Geometry: final body of the model. Coordinates: model frame, mm. A direction names the side the tool comes from. Coordinates: 2 decimals unless noted, no trailing zeros. Write each loop counter-clockwise with the first axis right and the second up, starting at its lowest first coordinate (ties: lowest second). Pieces come first, ordered by that corner, then holes.
from build123d import *

# Parameters (mm, degrees)
F0_W        = 2.5
F0_H        = 3.1
F0_W_2      = 3.1
F0_H_2      = 2.5
F1_DEPTH    = 15
F2_DEPTH    = 0.6
F3_T1_DEPTH = 15


# Not quite as in the source:
# - a fillet or chamfer that OpenCascade refuses, or shapes differently, is made with other operations: its cross-section is extruded or revolved along the edge and cut away or added


with BuildPart() as f1:
    # F0 (on Top) → F1 (new body)
    with BuildSketch(Plane.XY):
        with BuildLine():
            Line((39.1167589883, 43.6909709372), (38.9183741482, 43.5764333963))
            ThreePointArc((38.9183741482, 43.5764333963), (39.563732113, 42.8018800146), (40.1167589265, 41.9589202367))
            Line((40.1167589265, 41.9589202367), (39.1167589883, 43.6909709372))
        make_face()
        with BuildLine():
            ThreePointArc((40.1167589265, -41.8145826694), (39.563732113, -42.6575424473), (38.9183741482, -43.432095829))
            Line((38.9183741482, -43.432095829), (39.1167589883, -43.5466333699))
            Line((39.1167589883, -43.5466333699), (40.1167589265, -41.8145826694))
        make_face()
        with BuildLine():
            Line((41.1167589883, 40.226869322), (40.1167589265, 41.9589202367))
            ThreePointArc((40.1167589265, 41.9589202367), (40.5702701762, 41.0585049774), (40.9183741482, 40.1123317812))
            Line((40.9183741482, 40.1123317812), (41.1167589883, 40.226869322))
        make_face()
        with BuildLine():
            Line((41.1167589883, -40.0825317547), (40.9183741482, -39.9679942139))
            ThreePointArc((40.9183741482, -39.9679942139), (40.5702701762, -40.9141674102), (40.1167589265, -41.8145826694))
            Line((40.1167589265, -41.8145826694), (41.1167589883, -40.0825317547))
        make_face()
        with BuildLine():
            Line((38.9183741482, 43.5764333963), (23.9946357527, 34.9602090164))
            ThreePointArc((23.9946357527, 34.9602090164), (24.7962509126, 33.113620668), (25.9946357527, 31.4961074012))
            Line((25.9946357527, 31.4961074012), (40.9183741482, 40.1123317812))
            ThreePointArc((40.9183741482, 40.1123317812), (40.5702701762, 41.0585049774), (40.1167589265, 41.9589202367))
            ThreePointArc((40.1167589265, 41.9589202367), (39.563732113, 42.8018800146), (38.9183741482, 43.5764333963))
        make_face()
        with BuildLine():
            ThreePointArc((25.9946357527, -31.3517698339), (24.7962509126, -32.9692831007), (23.9946357527, -34.8158714491))
            Line((23.9946357527, -34.8158714491), (38.9183741482, -43.432095829))
            ThreePointArc((38.9183741482, -43.432095829), (39.563732113, -42.6575424473), (40.1167589265, -41.8145826694))
            ThreePointArc((40.1167589265, -41.8145826694), (40.5702701762, -40.9141674102), (40.9183741482, -39.9679942139))
            Line((40.9183741482, -39.9679942139), (25.9946357527, -31.3517698339))
        make_face()
        with BuildLine():
            Line((23.9946357527, 34.9602090164), (-12.8447652387, 13.6909709372))
            Line((-12.8447652387, 13.6909709372), (-20.6597652387, 27.2269479983))
            ThreePointArc((-20.6597652387, 27.2269479983), (-36.3375843281, 0.0721687836), (-20.6597652387, -27.082610431))
            Line((-20.6597652387, -27.082610431), (-12.8447652387, -13.5466333699))
            Line((-12.8447652387, -13.5466333699), (23.9946357527, -34.8158714491))
            ThreePointArc((23.9946357527, -34.8158714491), (24.7962509126, -32.9692831007), (25.9946357527, -31.3517698339))
            Line((25.9946357527, -31.3517698339), (25.7962509126, -31.2372322931))
            Line((25.7962509126, -31.2372322931), (25.7962509126, 31.3815698604))
            Line((25.7962509126, 31.3815698604), (25.9946357527, 31.4961074012))
            ThreePointArc((25.9946357527, 31.4961074012), (24.7962509126, 33.113620668), (23.9946357527, 34.9602090164))
        make_face()
        Polygon((-7.648612816, -11.9278312164), (-7.648612816, 12.0721687836), (21.7962509126, 29.0721687836), (21.7962509126, -28.9278312164), align=None, mode=Mode.SUBTRACT)
        Polygon((-17.998612816, 7.6721687836), (-11.648612816, 7.6721687836), (-11.648612816, 1.3221687836), (-11.648612816, -1.1778312164), (-11.648612816, -7.5278312164), (-17.998612816, -7.5278312164), (-20.498612816, -7.5278312164), (-26.848612816, -7.5278312164), (-26.848612816, -1.1778312164), (-26.848612816, 1.3221687836), (-26.848612816, 7.6721687836), (-20.498612816, 7.6721687836), align=None, mode=Mode.SUBTRACT)
        with Locations((-19.248612816, -5.9778312164)):
            Rectangle(F0_W, F0_H)
        with Locations((-13.198612816, 0.0721687836)):
            Rectangle(F0_W_2, F0_H_2)
        with Locations((-19.248612816, 6.1221687836)):
            Rectangle(F0_W, F0_H)
        with Locations((-25.298612816, 0.0721687836)):
            Rectangle(F0_W_2, F0_H_2)
    extrude(amount=F1_DEPTH)

    # F0 (on Top) → F2 (join)
    with BuildSketch(Plane.XY):
        with BuildLine():
            ThreePointArc((38.9183741482, 43.5764333963), (28.0338552197, 45.1965244366), (23.9946357527, 34.9602090164))
            Line((23.9946357527, 34.9602090164), (38.9183741482, 43.5764333963))
        make_face()
        with BuildLine():
            Line((39.1167589883, 43.6909709372), (38.9183741482, 43.5764333963))
            ThreePointArc((38.9183741482, 43.5764333963), (39.563732113, 42.8018800146), (40.1167589265, 41.9589202367))
            Line((40.1167589265, 41.9589202367), (39.1167589883, 43.6909709372))
        make_face()
        with BuildLine():
            Line((38.9183741482, -43.432095829), (23.9946357527, -34.8158714491))
            ThreePointArc((23.9946357527, -34.8158714491), (28.0338552197, -45.0521868693), (38.9183741482, -43.432095829))
        make_face()
        with BuildLine():
            ThreePointArc((40.1167589265, -41.8145826694), (39.563732113, -42.6575424473), (38.9183741482, -43.432095829))
            Line((38.9183741482, -43.432095829), (39.1167589883, -43.5466333699))
            Line((39.1167589883, -43.5466333699), (40.1167589265, -41.8145826694))
        make_face()
        with BuildLine():
            Line((41.1167589883, 40.226869322), (40.1167589265, 41.9589202367))
            ThreePointArc((40.1167589265, 41.9589202367), (40.5702701762, 41.0585049774), (40.9183741482, 40.1123317812))
            Line((40.9183741482, 40.1123317812), (41.1167589883, 40.226869322))
        make_face()
        with BuildLine():
            Line((40.9183741482, 40.1123317812), (25.9946357527, 31.4961074012))
            ThreePointArc((25.9946357527, 31.4961074012), (35.7032074646, 29.3083760539), (41.3018044121, 37.5362703988))
            ThreePointArc((41.3018044121, 37.5362703988), (41.2054217299, 38.8384907155), (40.9183741482, 40.1123317812))
        make_face()
        with BuildLine():
            ThreePointArc((41.3018044121, -37.3919328315), (35.7032074646, -29.1640384866), (25.9946357527, -31.3517698339))
            Line((25.9946357527, -31.3517698339), (40.9183741482, -39.9679942139))
            ThreePointArc((40.9183741482, -39.9679942139), (41.2054217299, -38.6941531482), (41.3018044121, -37.3919328315))
        make_face()
        with BuildLine():
            Line((41.1167589883, -40.0825317547), (40.9183741482, -39.9679942139))
            ThreePointArc((40.9183741482, -39.9679942139), (40.5702701762, -40.9141674102), (40.1167589265, -41.8145826694))
            Line((40.1167589265, -41.8145826694), (41.1167589883, -40.0825317547))
        make_face()
    extrude(amount=F2_DEPTH)

    # F3: fillet of radius 8 on 6 edges, made by hand

    # F3_s2 → F3_t1 (join)
    with BuildSketch(Plane.XY):
        with BuildLine():
            ThreePointArc((-3.648612816, 14.3815698604), (-6.5768160463, 11.4533666301), (-7.648612816, 7.4533666301))
            Line((-7.648612816, 7.4533666301), (-7.648612816, 12.0721687836))
            Line((-7.648612816, 12.0721687836), (-3.648612816, 14.3815698604))
        make_face()
        with BuildLine():
            ThreePointArc((25.7962509126, 26.7627677069), (26.8680476824, 30.7627677069), (29.7962509126, 33.6909709372))
            Line((29.7962509126, 33.6909709372), (25.7962509126, 31.3815698604))
            Line((25.7962509126, 31.3815698604), (25.7962509126, 26.7627677069))
        make_face()
        with BuildLine():
            ThreePointArc((21.7962509126, 15.2157623231), (17.7962509126, 22.1439655534), (9.7962509126, 22.1439655534))
            Line((9.7962509126, 22.1439655534), (21.7962509126, 29.0721687836))
            Line((21.7962509126, 29.0721687836), (21.7962509126, 15.2157623231))
        make_face()
        with BuildLine():
            ThreePointArc((21.7962509126, -15.0714247558), (17.7962509126, -21.9996279861), (9.7962509126, -21.9996279861))
            Line((9.7962509126, -21.9996279861), (21.7962509126, -28.9278312164))
            Line((21.7962509126, -28.9278312164), (21.7962509126, -15.0714247558))
        make_face()
        with BuildLine():
            ThreePointArc((29.7962509126, -33.5466333699), (26.8680476824, -30.6184301396), (25.7962509126, -26.6184301396))
            Line((25.7962509126, -26.6184301396), (25.7962509126, -31.2372322931))
            Line((25.7962509126, -31.2372322931), (29.7962509126, -33.5466333699))
        make_face()
        with BuildLine():
            ThreePointArc((-7.648612816, -7.3090290628), (-6.5768160463, -11.3090290628), (-3.648612816, -14.2372322931))
            Line((-3.648612816, -14.2372322931), (-7.648612816, -11.9278312164))
            Line((-7.648612816, -11.9278312164), (-7.648612816, -7.3090290628))
        make_face()
    extrude(amount=F3_T1_DEPTH)


solid = f1.part
Item 1: Pin query (flat end, axial travel): pin 1 (1 mm diameter, centred on x = 23.5, z = 3, fed in from +Y); pin 2 (0.8 mm diameter, centred on x = -19, z = 6, fed in from -Y); pin 3 (1.9 mm diameter, centred on y = 5.5, z = 5, fed in from +X). Return the tip coordinate at first contact, or that it passes through.
Derived:
pin 1: stops at y = 34.96
pin 2: stops at y = -24.9
pin 3: stops at x = 25.8
Item 2: Pull-direction query (Y, two-part tool) for faces 1 (the flat face through (29, 42, 0.6)), 2 (the flat face through (-23.749, 0, 7)), 3 (the flat face through (2.98, 18.21, 7.4)), 4 (the flat face through (-16.8, -20.4, 7.4)); classes: released by +Y, released by -Y, zero draft, split by the parting line, or undercut.
Derived:
face 1: zero draft
face 2: undercut
face 3: undercut
face 4: released by -Y
Item 3: Material intervals for probe 1 along Y at (x, z) = (-26, 2.25); probe 2 along X at (y, z) = (-16, 14.25); probe 3 along X at (y, z) = (-7, 5.75), sorted ascending.
Derived:
probe 1: y = -23.2 to -7.53, -1.18 to 1.32, 7.67 to 23.34
probe 2: x = -31.91 to -14.26, -8.6 to -0.6, 21.74 to 25.8
probe 3: x = -35.53 to -26.85, -20.5 to -18, -11.65 to -7.65, 21.8 to 25.8
Item 4: Section D-D, the plane y = -6. Output: boundary loops of the cut face in (x, z), plus the area to 3 significant figures.
Derived:
outline: (-35.74, 0) - (-26.85, 0) - (-26.85, 15) - (-35.74, 15) - close; (-20.5, 0) - (-18, 0) - (-18, 15) - (-20.5, 15) - close; (-11.65, 0) - (-7.65, 0) - (-7.65, 15) - (-11.65, 15) - close; (21.8, 0) - (25.8, 0) - (25.8, 15) - (21.8, 15) - close
area: 291 mm2
Item 5: Section B-B, the plane x = 16. Output: boundary loops of the cut face in (y, z).
Derived:
outline: (-30.2, 0) - (-22.76, 0) - (-22.76, 15) - (-30.2, 15) - close; (22.91, 0) - (30.34, 0) - (30.34, 15) - (22.91, 15) - close
Item 6: Set-up query: faces 5 (the flat face through (36, 33, 0.6)), 6 (the cylindrical face through (-36.334, 0.532, 7.395)), 7 (the flat face through (25.796, 0, 7)), 8 (the cylindrical face through (17.9, -21.94, 7.4)). Return all of +Z, -Z, +X, -X, +Y, -Y with unobstructed straight access to the full face (end or side cutting, diameter ignored); none if empty.
Derived:
face 5: +Z, +X
face 6: +Z, -Z, -X
face 7: +Z, -Z, +X
face 8: +Z, -Z
Item 7: Section A-A, the plane y = -20. Output: boundary loops of the cut face in (x, z), plus the area to 3 significant figures.
Derived:
outline: (-29.07, 0) - (-16.57, 0) - (-16.57, 15) - (-29.07, 15) - close; (-1.67, 0) - (6.33, 0) - (6.33, 15) - (-1.67, 15) - close; (20.1, 0) - (25.8, 0) - (25.8, 15) - (20.1, 15) - close
area: 393 mm2
Item 8: Section C-C, the plane z = 12. State how many separate pieces and enclosed holes the cut face has, plus the area to 3 significant figures.
Derived:
separate pieces: 1
enclosed holes: 2
area: 1,660 mm2
